from build123d import *

# Parameters (mm, degrees)
SKETCH_1_R      = 11
SKETCH_1_R_2    = 2.1
EXTRUDE_1_DEPTH = 3
FILLET_1_R      = 5


with BuildPart() as part:
    # ｽｹｯﾁ1 → ﾎﾞｽ - 押し出し1 (new body)
    with BuildSketch(Plane.XY):
        with BuildLine():
            Line((-40, 22.5), (0, 22.5))
            ThreePointArc((0, 22.5), (22.5, 0), (0, -22.5))
            Line((0, -22.5), (-40, -22.5))
            Line((-40, -22.5), (-50, -22.5))
            Line((-50, -22.5), (-50, 22.5))
            Line((-50, 22.5), (-40, 22.5))
        make_face()
        Circle(SKETCH_1_R, mode=Mode.SUBTRACT)
        with Locations((-45, 17.5)):
            Circle(SKETCH_1_R_2, mode=Mode.SUBTRACT)
        with Locations(Location((-45, -17.5, 0), (0, 0, 180))):
            Circle(SKETCH_1_R_2, mode=Mode.SUBTRACT)
    extrude(amount=EXTRUDE_1_DEPTH)

    # ﾌｨﾚｯﾄ1
    fillet_1_edges = [part.edges().sort_by_distance(p)[0] for p in [
        (-50, -22.5, 1.5),
        (-50, 22.5, 1.5),
    ]]
    fillet(fillet_1_edges, radius=FILLET_1_R)


solid = part.part
Here's how the part is built. I have some questions about the finished solid (model axes, mm). Coordinates: 2 decimals unless noted, no trailing zeros. Order: outer loops, then holes, each group sorted by start corner. A loop starts at its lowest first (then second) coordinate and runs counter-clockwise, first axis right, second up. Notation, with made-up numbers: M -5,89 L 19,89 A28 cw 19,108 Z; hole C 69.25,18.25 d9. An arc over 180 degrees is marked long. Answer as CSV lines item,"result".
Item 1: Imagine slicing it at D-D on x = 17. Write out the boundary of the cut face in (y, z), plus the area to 3 significant figures.
Results found:
outline,"M -14.74,0 L 14.74,0 L 14.74,3 L -14.74,3 Z"
area,"88.4 mm2"
Item 2: For pin 1 (1 mm diameter, centred on x = 9.5, z = 2, fed in from -Y), with a flat end and sliding along its axis, tell me the tip position at first contact or that it passes through.
Results found:
pin 1,"y = -20.62"
Item 3: Imagine slicing it at A-A on z = 2.2. Write out the boundary of the cut face in (x, y).
Results found:
outline,"M -50,-17.5 A5 ccw -45,-22.5 L 0,-22.5 A22.5 ccw 0,22.5 L -45,22.5 A5 ccw -50,17.5 Z; hole C -45,-17.5 d4.2; hole C -45,17.5 d4.2; hole C 0,0 d22"
Item 4: Imagine slicing it at C-C on x = 9. Write out the boundary of the cut face in (y, z), plus the area to 3 significant figures.
Results found:
outline,"M -20.62,0 L -6.32,0 L -6.32,3 L -20.62,3 Z; M 6.32,0 L 20.62,0 L 20.62,3 L 6.32,3 Z"
area,"85.8 mm2"
Item 5: If I drill on line 1 (Y direction, x = -45, z = 1.85); line 2 (Y direction, x = -44.5, z = 0.55); line 3 (X direction, y = 2.5, z = 2.2), over which ranges is the centre line in solid material (lowest first)?
Results found:
line 1,"-22.5 to -19.6, -15.4 to 15.4, 19.6 to 22.5"
line 2,"-22.5 to -19.54, -15.46 to 15.46, 19.54 to 22.5"
line 3,"-50 to -10.71, 10.71 to 22.36"
Item 6: We'd pull the mould along X, two halves only. Please class faces 1 (the face through (-22, -22.5, 1)), 2 (the face through (-50, 0, 1)), 3 (the face through (-46.13, -19.27, 1.48)): +X half, -X half, draft (parallel to the pull), parting line (faces both ways), or undercut.
Results found:
face 1,"draft"
face 2,"-X half"
face 3,"undercut"
Item 7: Imagine slicing it at B-B on y = 0. Write out the boundary of the cut face in (x, z), plus the area to 4 significant figures.
Results found:
outline,"M -50,0 L -11,0 L -11,3 L -50,3 Z; M 11,0 L 22.5,0 L 22.5,3 L 11,3 Z"
area,"151.5 mm2"
